```python
from build123d import *

# Parameters (mm, degrees)
SKETCH_1_W          = 32
SKETCH_1_H          = 12.5
EXTRUDE_1_DEPTH     = 23
SKETCH_3_W          = 4.75
SKETCH_3_H          = 12.5
CUT_EXTRUDE_2_DEPTH = 4
SKETCH_8_W          = 4.75
SKETCH_8_H          = 12.5
CUT_EXTRUDE_3_DEPTH = 16.1
SKETCH_9_R          = 3
EXTRUDE_2_DEPTH     = 3
SKETCH_10_R         = 1.356770986
EXTRUDE_3_DEPTH     = 5


with BuildPart() as part:
    # 草图1 → 凸台-拉伸1 (new body)
    with BuildSketch(Plane(origin=(0, 0, 0), x_dir=(1, 0, 0), z_dir=(0, 1, 0))):
        Rectangle(SKETCH_1_W, SKETCH_1_H)
    extrude(amount=EXTRUDE_1_DEPTH)

    # 草图3 → 切除-拉伸2 (cut)
    with BuildSketch(Plane(origin=(0, 23, 0), x_dir=(1, 0, 0), z_dir=(0, 1, 0))):
        with Locations((-13.625, 0)):
            Rectangle(SKETCH_3_W, SKETCH_3_H)
        with Locations((13.625, 0)):
            Rectangle(SKETCH_3_W, SKETCH_3_H)
    extrude(amount=-CUT_EXTRUDE_2_DEPTH, mode=Mode.SUBTRACT)

    # 草图8 → 切除-拉伸3 (cut)
    with BuildSketch(Plane.XZ):
        with Locations((13.625, 0)):
            Rectangle(SKETCH_8_W, SKETCH_8_H)
        with Locations((-13.625, 0)):
            Rectangle(SKETCH_8_W, SKETCH_8_H)
    extrude(amount=-CUT_EXTRUDE_3_DEPTH, mode=Mode.SUBTRACT)

    # 草图9 → 凸台-拉伸2 (add)
    with BuildSketch(Plane(origin=(0, 23, 0), x_dir=(1, 0, 0), z_dir=(0, 1, 0))):
        with Locations(Location((7.766955593, 0, 0), (0, 0, 270))):
            Circle(SKETCH_9_R)
    extrude(amount=EXTRUDE_2_DEPTH)

    # 草图10 → 凸台-拉伸3 (add)
    with BuildSketch(Plane(origin=(0, 26, 0), x_dir=(1, 0, 0), z_dir=(0, 1, 0))):
        with Locations(Location((7.766955593, 0, 0), (0, 0, 270))):
            Circle(SKETCH_10_R)
    extrude(amount=EXTRUDE_3_DEPTH)


solid = part.part
```
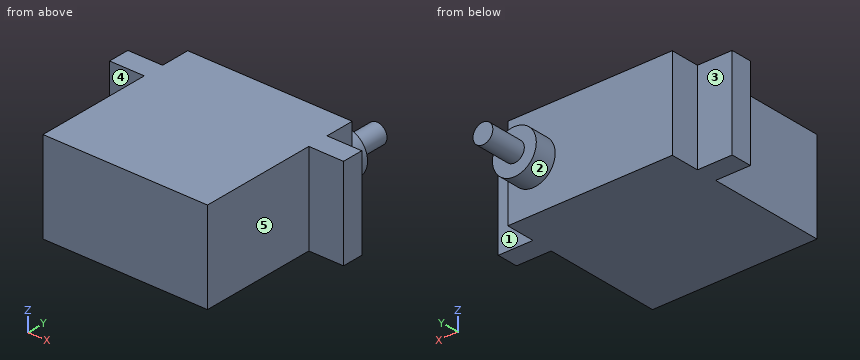
Can you work these out from the model? Positions are in its coordinate system, mm. Face numbers are marked on the shaded views. A direction names the side the tool comes from. Coordinates: 2 decimals unless noted, no trailing zeros. Loops run counter-clockwise (first coordinate to the right, second up) from the corner with the lowest first, then second, coordinate; pieces in that order, holes last.
1) I need wall thicknesses on probe 1 along X at (y, z) = (10, 1.25); probe 2 along Y at (x, z) = (0.5, -3); probe 3 along Y at (x, z) = (6, 0.5). Which ranges of each line are inside material? Lowest first, please.
2) Imagine slicing it at C-C on y = 5. List the corners of the cut face in (x, z) for me.
3) Imagine slicing it at B-B on x = 5.5. List the corners of the cut face in (y, z) for me.
4) Imagine slicing it at D-D on z = 0. List the corners of the cut face in (x, y) for me, plus the area to 3 significant figures.
5) Imagine slicing it at A-A on z = -5.25. List the corners of the cut face in (x, y) for me, plus the area to 3 significant figures.
6) Which directions (+Z, -Z, +X, -X, +Y, -Y) give clear straight access to the entire face, cutting with the end or side of a thin tool? Please do the marked faces 1, 2, 3, 4 and 5.
7) For pin 1 (6 mm diameter, centred on y = 5.5, z = 2, fed in from -X); pin 2 (4 mm diameter, centred on y = 25.5, z = 2, fed in from +X); pin 3 (2.5 mm diameter, centred on x = 14.5, z = -1.5, fed in from +Y); pin 4 (1 mm diameter, centred on x = 4.5, z = -1.5, fed in from -Y), each with a flat end and sliding along its axis, tell me the tip position at first contact or that it passes through.
Completed:
1. probe 1: x = -11.25 to 11.25
1. probe 2: y = 0 to 23
1. probe 3: y = 0 to 26
2. outline: (-11.25, -6.25) - (11.25, -6.25) - (11.25, 6.25) - (-11.25, 6.25) - close
3. outline: (0, -6.25) - (23, -6.25) - (23, -1.96) - (26, -1.96) - (26, 1.96) - (23, 1.96) - (23, 6.25) - (0, 6.25) - close
4. outline: (-16, 16.1) - (-11.25, 16.1) - (-11.25, 0) - (11.25, 0) - (11.25, 16.1) - (16, 16.1) - (16, 19) - (11.25, 19) - (11.25, 23) - (10.77, 23) - (10.77, 26) - (9.12, 26) - (9.12, 31) - (6.41, 31) - (6.41, 26) - (4.77, 26) - (4.77, 23) - (-11.25, 23) - (-11.25, 19) - (-16, 19) - close
4. area: 577 mm2
5. outline: (-16, 16.1) - (-11.25, 16.1) - (-11.25, 0) - (11.25, 0) - (11.25, 16.1) - (16, 16.1) - (16, 19) - (11.25, 19) - (11.25, 23) - (-11.25, 23) - (-11.25, 19) - (-16, 19) - close
5. area: 545 mm2
6. face 1: +Z, -Z, +X, +Y
6. face 2: +Y
6. face 3: +Z, -Z, -X, +Y
6. face 4: +Z, -Z, -X, -Y
6. face 5: +Z, -Z, +X, -Y
7. pin 1: stops at x = -11.25
7. pin 2: stops at x = 10.77
7. pin 3: stops at y = 19
7. pin 4: stops at y = 0
